Geometry: see drawing. Coordinates: mm, zero at the bounding-box minimum. A direction names the side the tool comes from. Coordinates: 2 decimals unless noted, no trailing zeros. Order: outer loops, then holes, each group sorted by start corner. A loop starts at its lowest first (then second) coordinate and runs counter-clockwise, first axis right, second up. Notation, with made-up numbers: (-9.5, 80.5) -> (14.5, 80.5) arc R20 cw to (14.5, 93.5) -> close; hole circle Ø4 at (8.5, 29). An arc over 180 degrees is marked (long way). Use one line per item in the form item = value.
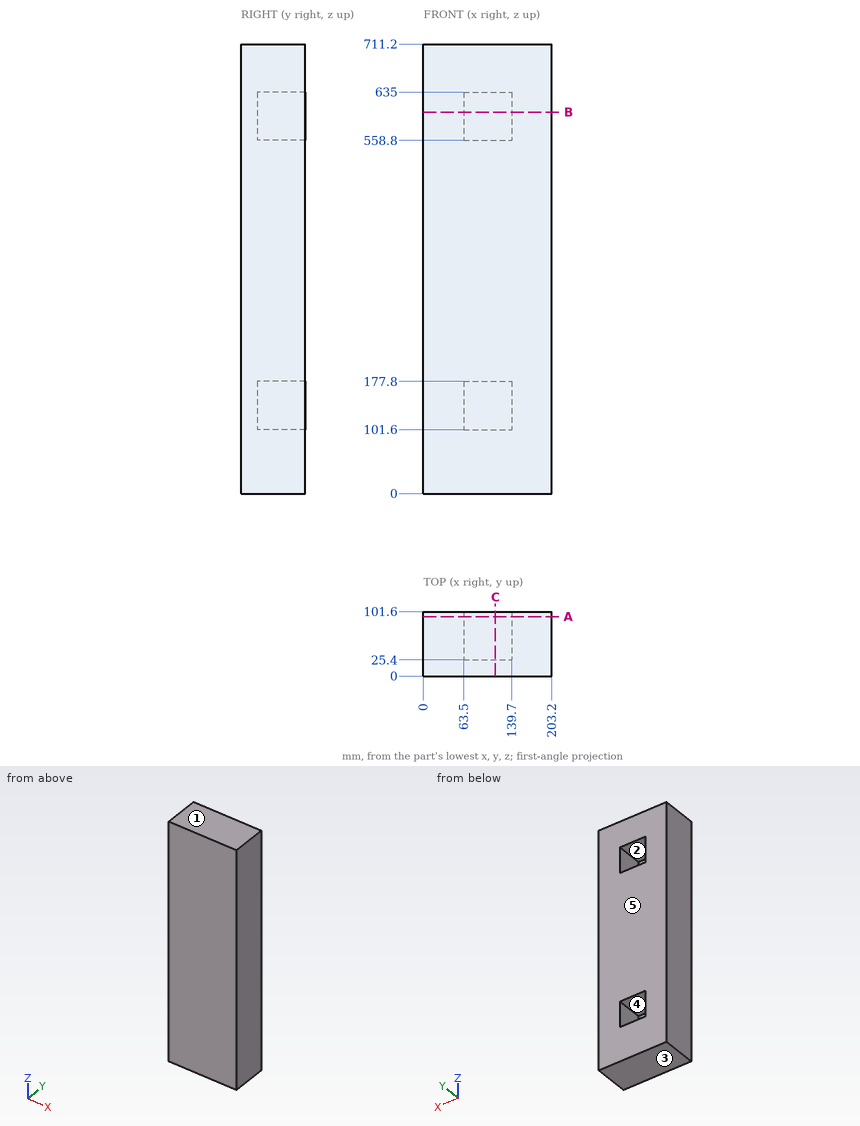
1) Section A-A, the plane y = 94. Output: boundary loops of the cut face in (x, z), and give its area (3 significant figures).
Results found:
outline = (0, 0) -> (203.2, 0) -> (203.2, 711.2) -> (0, 711.2) -> close; hole (63.5, 101.6) -> (139.7, 101.6) -> (139.7, 177.8) -> (63.5, 177.8) -> close; hole (63.5, 558.8) -> (139.7, 558.8) -> (139.7, 635) -> (63.5, 635) -> close
area = 133,000 mm2
2) Contact query for a flat-ended pin moving along its axis: P1, Ø23, axis at x = 84, z = 158.5, coming from the +Y side. Output: stop coordinate, or through.
Results found:
P1 = 25.4
3) Section B-B, the plane z = 603.5. Output: boundary loops of the cut face in (x, y).
Results found:
outline = (0, 0) -> (203.2, 0) -> (203.2, 101.6) -> (139.7, 101.6) -> (139.7, 25.4) -> (63.5, 25.4) -> (63.5, 101.6) -> (0, 101.6) -> close
4) Pull-direction query (Z, two-part tool) for the marked faces 3, 4 and 5; classes: released by +Z, released by -Z, zero draft, split by the parting line, or undercut.
Results found:
face_3 = released by -Z
face_4 = undercut
face_5 = zero draft
5) Access query for the marked faces 1 and 2. Directions: +Z, -Z, +X, -X, +Y, -Y. A direction counts if a zero-diameter tool reaches every point of the face in a straight line with its end or side. Return the directions, or none.
Results found:
face_1 = +Z, +X, -X, +Y, -Y
face_2 = +Y
6) Section C-C, the plane x = 114. Output: boundary loops of the cut face in (y, z), and give its area (3 significant figures).
Results found:
outline = (0, 0) -> (101.6, 0) -> (101.6, 101.6) -> (25.4, 101.6) -> (25.4, 177.8) -> (101.6, 177.8) -> (101.6, 558.8) -> (25.4, 558.8) -> (25.4, 635) -> (101.6, 635) -> (101.6, 711.2) -> (0, 711.2) -> close
area = 60,600 mm2
7) Material intervals for probe 1 along Z at (x, y) = (74, 92); probe 2 along X at (y, z) = (86, 153.5); probe 3 along Y at (x, z) = (90.5, 619.5), sorted ascending. Write a range as from..to.
Results found:
probe_1 = 0..101.6, 177.8..558.8, 635..711.2
probe_2 = 0..63.5, 139.7..203.2
probe_3 = 0..25.4
